from build123d import *

# Parameters (mm, degrees)
SKETCH1_W           = 55.88
SKETCH1_H           = 44.45
BOSS_EXTRUDE1_DEPTH = 3.175
SKETCH2_W           = 62.23
SKETCH2_H           = 50.8
SKETCH2_W_2         = 55.88
SKETCH2_H_2         = 44.45
BOSS_EXTRUDE2_DEPTH = 7.62
FILLET1_R           = 2.54
SKETCH4_R           = 5.08
CUT_EXTRUDE1_DEPTH  = 15.875


with BuildPart() as part:
    # Sketch1 → Boss-Extrude1 (new body)
    with BuildSketch(Plane.XY):
        Rectangle(SKETCH1_W, SKETCH1_H)
    extrude(amount=BOSS_EXTRUDE1_DEPTH)

    # Sketch2 → Boss-Extrude2 (add)
    with BuildSketch(Plane.XY.offset(3.175)):
        Rectangle(SKETCH2_W, SKETCH2_H)
        Rectangle(SKETCH2_W_2, SKETCH2_H_2, mode=Mode.SUBTRACT)
    extrude(amount=-BOSS_EXTRUDE2_DEPTH)

    # Sketch3 → Revolve1 (revolve)
    with BuildSketch(Plane(origin=(0, 0, 0), x_dir=(1, 0, 0), z_dir=(0, 1, 0)), mode=Mode.PRIVATE) as revolve1_sk:
        with BuildLine():
            Line((0, -3.175), (6.35, -3.175))
            Line((6.35, -3.175), (6.35, -10.331555752))
            ThreePointArc((6.35, -10.331555752), (25.197554285, -38.125509029), (0, -60.325))
            Line((0, -60.325), (0, -3.175))
        make_face()
    revolve(revolve1_sk.sketch.rotate(Axis((0, 0, 0), (0, 0, 1)), 180), axis=Axis((0, 0, 0), (0, 0, 1)))

    # Fillet1
    fillet1_edges = [part.edges().sort_by_distance(p)[0] for p in [
        (6.35, 0, 3.175),
        (6.35, 0, 10.331555752),
    ]]
    fillet(fillet1_edges, radius=FILLET1_R)

    # Sketch4 → Cut-Extrude1 (cut)
    with BuildSketch(Plane.XY.offset(3.175)):
        with Locations((-20.955, 0)):
            Circle(SKETCH4_R)
    extrude(amount=-CUT_EXTRUDE1_DEPTH, mode=Mode.SUBTRACT)


solid = part.part
Design review of the part built by this model. Coordinates are the model's own, in mm. A direction names the side the tool comes from. Give positions to 0.01 mm unless a question says otherwise; leave off trailing zeros. Write each loop counter-clockwise with the first axis right and the second up, starting at its lowest first coordinate (ties: lowest second). Pieces come first, ordered by that corner, then holes. Notation, with made-up numbers: M -19.75,86 L 5.25,86 A20 ccw 5.25,111 Z; hole C 10,10 d2. An arc over 180 degrees is marked long. Return JSON: item names as keys, results as strings. Group by question number.
Item 1: Take a section at C-C (z = 21). Give the boundary of the cut face in (x, y).
Item 2: Take a section at D-D (z = 34). Give the boundary of the cut face in (x, y), plus the area to 3 significant figures.
Item 3: Take a section at B-B (x = 13.5). Give the boundary of the cut face in (y, z) (3 decimals).
Item 4: The part is to be moulded in two halves that separate along Y. For faces 4 (the flat face through (-27.94, 0, -2)), 5 (the flat face through (0, -22.225, -2)), 6 (the cylindrical face through (-6.057, -1.907, 7.095)), 7 (the flat face through (-2.5, -22.5, -4.445)), say which applies: pulls with the +Y half, pulls with the -Y half, needs draft (parallel to the pull), parting line crosses it, or undercut.
Item 5: Wall thickness on line 1 along X through (y, z) = (5, -2) (3 decimals); line 2 along Z through (x, y) = (14, 2.5) (3 decimals); line 3 along Z through (x, y) = (-7.5, -15) (3 decimals): over which ranges is each line inside the solid? List them lowest first.
Item 6: Tool access review of faces 1 (the flat face through (0, -25.4, -1)), 2 (the flat face through (-7, 6, 3.175)), 3 (the flat face through (27.94, 0, -2)): name each direction out of +Z, -Z, +X, -X, +Y, -Y from which nothing blocks a thin tool from reaching the whole face with its end or side.
Item 7: Clearance check with flat-ended pins moving along their axes: pin 1 Ø9 at (x, y) = (-20.955, 0) entering from +Z; pin 2 Ø12 at (y, z) = (2, 43.5) entering from -X; pin 3 Ø10 at (y, z) = (-10.5, 24.5) entering from -X. State where each tip first meets the part, or that it passes through.
Item 8: Take a section at A-A (y = 17). Give the boundary of the cut face in (x, z) (3 decimals).
Return value:
{
 "1": {"outline": "C 0,0 d42.49"},
 "2": {"outline": "C 0,0 d50.77", "area": "2,020 mm2"},
 "3": {"outline": "M -25.4,-4.445 L -22.225,-4.445 L -22.225,0 L 22.225,0 L 22.225,-4.445 L 25.4,-4.445 L 25.4,3.175 L -25.4,3.175 Z; C 0,34.925 d43.031"},
 "4": {"face 4": "undercut", "face 5": "undercut", "face 6": "parting line crosses it", "face 7": "needs draft"},
 "5": {"line 1": "x = -31.115 to -27.94, 27.94 to 31.115", "line 2": "z = 0 to 3.175, 13.88 to 55.97", "line 3": "z = 0 to 3.175, 15.849 to 54.001"},
 "6": {"face 1": "+Z, -Z, +X, -X, -Y", "face 2": "none", "face 3": "-Z"},
 "7": {"pin 1": "stops at z = 54.27", "pin 2": "stops at x = -25.24", "pin 3": "stops at x = -23.43"},
 "8": {"outline": "M -31.115,-4.445 L -27.94,-4.445 L -27.94,0 L 27.94,0 L 27.94,-4.445 L 31.115,-4.445 L 31.115,3.175 L -31.115,3.175 Z; C 0,34.925 d37.744"}
}
